Check sheet for the modelled part. Datum: model origin and axes. Units: mm. Face numbers are marked on the shaded views. Coordinates: 2 decimals unless noted, no trailing zeros. Order: outer loops, then holes, each group sorted by start corner. A loop starts at its lowest first (then second) coordinate and runs counter-clockwise, first axis right, second up.
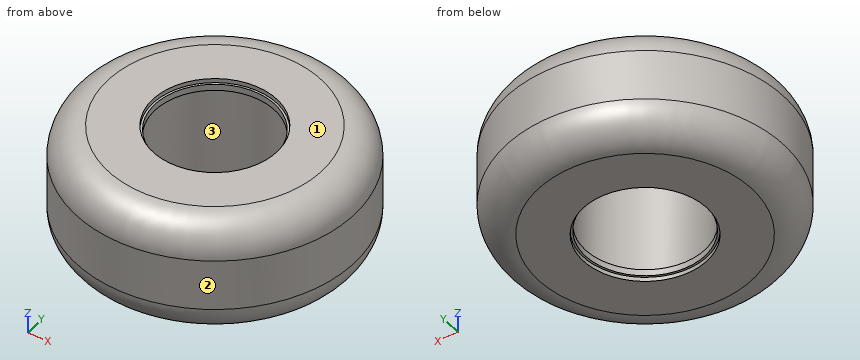
from build123d import *

# Parameters (mm, degrees)
SKETCH_1_R          = 65
SKETCH_1_R_2        = 28
EXTRUDE_1_DEPTH     = 54
SKETCH_2_R          = 29
CUT_EXTRUDE_1_DEPTH = 2
CUT_EXTRUDE_START   = -2
SKETCH_3_R          = 29
CUT_EXTRUDE_2_DEPTH = 2
SKETCH_4_W          = 1
SKETCH_4_H          = 44
FILLET_1_R          = 15


with BuildPart() as part:
    # 草图1 → 凸台-拉伸1 (new body)
    with BuildSketch(Plane.XY):
        Circle(SKETCH_1_R)
        Circle(SKETCH_1_R_2, mode=Mode.SUBTRACT)
    extrude(amount=EXTRUDE_1_DEPTH)

    # 草图2 → 切除-拉伸1 (cut)
    with BuildSketch(Plane(origin=(0, 0, 0), x_dir=(-1, 0, 0), z_dir=(0, 0, -1))):
        Circle(SKETCH_2_R)
    extrude(amount=-CUT_EXTRUDE_1_DEPTH, mode=Mode.SUBTRACT)

    # 草图3 → 切除-拉伸2 (cut)
    with BuildSketch(Plane.XY.offset(54).offset(CUT_EXTRUDE_START)):
        with Locations(Location((0, 0, 0), (0, 0, 180))):
            Circle(SKETCH_3_R)
    extrude(amount=CUT_EXTRUDE_2_DEPTH, mode=Mode.SUBTRACT)

    # 草图4 → 切除-旋转1 (revolve, cut)
    with BuildSketch(Plane(origin=(0, 0, 0), x_dir=(1, 0, 0), z_dir=(0, 1, 0))):
        with Locations((-28.017381105, -27)):
            Rectangle(SKETCH_4_W, SKETCH_4_H)
    revolve(axis=Axis((0, 0, 0), (0, 0, 1)), mode=Mode.SUBTRACT)

    # 圆角1
    fillet_1_edges = [part.edges().sort_by_distance(p)[0] for p in [
        (-65, 0, 0),
        (-65, 0, 54),
    ]]
    fillet(fillet_1_edges, radius=FILLET_1_R)


solid = part.part
(1) Release check for a two-part mould opening along Z. For the marked faces 1, 2 and 3 record: +Z half, -Z half, draft (parallel to the pull), parting line (faces both ways), or undercut.
Filled in:
face 1: +Z half
face 2: draft
face 3: undercut
(2) Cross-section at A-A (x = 0). Enter the section's corners in (y, z).
Filled in:
outline: (-65, 15) arc R15 ccw to (-50, 0) - (-29, 0) - (-29, 2) - (-28, 2) - (-28, 5) - (-28.52, 5) - (-28.52, 49) - (-28, 49) - (-28, 52) - (-29, 52) - (-29, 54) - (-50, 54) arc R15 ccw to (-65, 39) - close; (28, 2) - (29, 2) - (29, 0) - (50, 0) arc R15 ccw to (65, 15) - (65, 39) arc R15 ccw to (50, 54) - (29, 54) - (29, 52) - (28, 52) - (28, 49) - (28.52, 49) - (28.52, 5) - (28, 5) - close
(3) Cross-section at C-C (z = 26.5). Enter the section's corners in (x, y).
Filled in:
outline: circle Ø130 at (0, 0); hole circle Ø57.03 at (0, 0)
(4) Thickness scan on probe 1 along Y at (x, z) = (0, 33); probe 2 along Z at (x, y) = (44, 24.5); probe 3 along X at (y, z) = (-15, 31.5). Record the ranges inside material, lowest first.
Filled in:
probe 1: y = -65 to -28.52, 28.52 to 65
probe 2: z = 0 to 54
probe 3: x = -63.25 to -24.25, 24.25 to 63.25
(5) Go/stop test with flat-tipped pins: P1, Ø4, axis at x = 45, z = 28, coming from the -Y side; P2, Ø8, axis at y = -38.5, z = 28, coming from the -X side; P3, Ø10, axis at x = -49.5, z = 5.5, coming from the -Y side; P4, Ø3, axis at x = -47.5, y = -47, coming from the +Z side. Record where each tip stops, or that it passes through.
Filled in:
P1: stops at y = -48.74
P2: stops at x = -55.09
P3: stops at y = -44.33
P4: passes through
